from build123d import *

# Parameters (mm, degrees)
F2_SIZE        = 3.175
F3_R           = 0.254
F6_D           = 5.1054
F6_DEPTH       = 49.3522
F6_START       = 0.2754562
F6_CBORE_D     = 10.414
F6_CBORE_DEPTH = 33.4772
F6_TIP         = 1.5338169022


# Not quite as in the source:
# - a feature names something its author has since deleted; it is built from what else it names


with BuildPart() as f1:
    # F0 (on Right) → F1 (revolve)
    with BuildSketch(Plane.YZ):
        Polygon((-41.4782, 10.0076), (0, 10.0076), (41.4782, 10.0076), (41.4782, 49.3522), (13.1445, 49.3522), (13.1445, 23.5712), (9.7155, 23.5712), (9.7155, 44.8818), (-13.1445, 44.8818), (-13.1445, 49.3522), (-41.4782, 49.3522), align=None)
    revolve(axis=Axis((0, -0.9843776588, 0), (0, 1, 0)))

    # F2
    f2_edges = [f1.edges().sort_by_distance(p)[0] for p in [
        (0, 9.7155, -44.8818),
    ]]
    chamfer(f2_edges, length=F2_SIZE)

    # F3
    f3_edges = [f1.edges().sort_by_distance(p)[0] for p in [
        (0, 9.7155, -23.5712),
        (0, 13.1445, -23.5712),
    ]]
    fillet(f3_edges, radius=F3_R)

    # F6
    # its depths count from where the whole tool has entered the part; down to there all is cleared
    with Locations(Plane.XY.offset(49.3522).offset(-F6_START)):
        with Locations((0, 36.2458)):
            CounterBoreHole(F6_D / 2, F6_CBORE_D / 2, F6_CBORE_DEPTH, depth=F6_DEPTH)
            with Locations((0, 0, -(F6_DEPTH + F6_TIP / 2))):  # 118° drill point
                Cone(0, F6_D / 2, F6_TIP, mode=Mode.SUBTRACT)


solid = f1.part
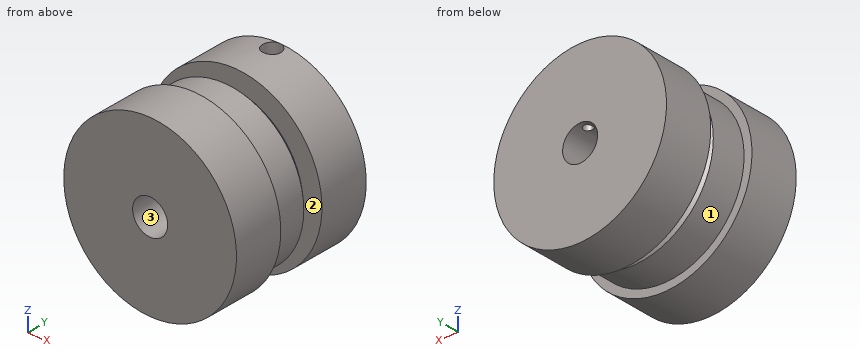
Geometry check sheet. Reference: the model listing, model coordinates, mm. Face numbers are marked on the shaded views. Coordinates: 2 decimals unless noted, no trailing zeros. Order: outer loops, then holes, each group sorted by start corner. A loop starts at its lowest first (then second) coordinate and runs counter-clockwise, first axis right, second up. Notation, with made-up numbers: (-2.5, 59) -> (21.5, 59) arc R22 cw to (21.5, 84) -> close; hole circle Ø2 at (-39.5, 83). An arc over 180 degrees is marked (long way). Use a Markdown table: item, result. Add a question column.
1. Cross-section at A-A (x = 0). Give the number of separate pieces and of enclosed holes in the cut face, and give its area (3 significant figures).
2. Cross-section at B-B (z = 0). Enter the section's corners in (x, y).
3. Material ranges on L1, parallel to Y at x = 16.5, z = 27; L2, parallel to Y at x = 0, z = 12.65; L3, parallel to Z at x = -4, y = 21, recorded low to high.
4. Mould release check, pull along Z, two halves, no side actions. Record for the marked faces 1, 2 and 3: pulls with the +Z half, pulls with the -Z half, needs draft (parallel to the pull), parting line crosses it, or undercut.
5. Go/stop test with flat-tipped pins: pin 1 Ø2 at (x, y) = (-39.5, 32.5) entering from +Z; pin 2 Ø4 at (x, y) = (0, 36.25) entering from +Z; pin 3 Ø1.5 at (y, z) = (31.5, 22.5) entering from -X. Record where each tip stops, or that it passes through.
6. Cross-section at C-C (y = -16). Enter the section's corners in (x, z).
Filled sheet:
| question | item | result |
|---|---|---|
| 1 | separate pieces | 3 |
| 1 | enclosed holes | 0 |
| 1 | area | 5,760 mm2 |
| 2 | outline | (-49.35, -41.48) -> (-10.01, -41.48) -> (-10.01, 41.48) -> (-49.35, 41.48) -> (-49.35, 13.14) -> (-23.83, 13.14) arc R0.25 cw to (-23.57, 12.89) -> (-23.57, 9.97) arc R0.25 cw to (-23.83, 9.72) -> (-41.71, 9.72) -> (-44.88, 6.54) -> (-44.88, -13.14) -> (-49.35, -13.14) -> close; (10.01, -41.48) -> (49.35, -41.48) -> (49.35, -13.14) -> (44.88, -13.14) -> (44.88, 6.54) -> (41.71, 9.72) -> (23.83, 9.72) arc R0.25 cw to (23.57, 9.97) -> (23.57, 12.89) arc R0.25 cw to (23.83, 13.14) -> (49.35, 13.14) -> (49.35, 41.48) -> (10.01, 41.48) -> close |
| 3 | L1 | -41.48 to 9.72, 13.14 to 41.48 |
| 3 | L2 | -41.48 to 33.69, 38.8 to 41.48 |
| 3 | L3 | -49.19 to -9.17, 9.17 to 49.19 |
| 4 | face 1 | parting line crosses it |
| 4 | face 2 | needs draft |
| 4 | face 3 | undercut |
| 5 | pin 1 | z = 30.88 |
| 5 | pin 2 | z = -9.81 |
| 5 | pin 3 | x = -44.3 |
| 6 | outline | circle Ø98.7 at (0, 0); hole circle Ø20.02 at (0, 0) |
